from build123d import *

# Parameters (mm, degrees)
F1_W     = 43.7
F1_H     = 42.4
F1_R     = 1.5
F1_W_2   = 5
F1_H_2   = 4.4
F2_DEPTH = 1
F3_SIZE  = 0.99999
F4_DEPTH = 1
F5_W     = 19
F5_H     = 1
F6_DEPTH = 12


# Not quite as in the source:
# - a fillet or chamfer is up to 0.001 mm smaller than in the source, because OpenCascade refuses the exact size


with BuildPart() as f2:
    # F1 (on face) → F2 (new body)
    with BuildSketch(Plane.XY):
        with Locations((-38.7602308843, 29.1194021702)):
            Rectangle(F1_W, F1_H)
        with Locations((-53.3102308843, 12.9194021702)):
            Circle(F1_R, mode=Mode.SUBTRACT)
        with Locations((-48.3102308843, 13.1194021702)):
            Circle(F1_R, mode=Mode.SUBTRACT)
        with Locations((-41.9102308843, 33.1194021702)):
            Rectangle(F1_W_2, F1_H_2, mode=Mode.SUBTRACT)
        with Locations((-30.4102308843, 38.3194021702)):
            Circle(F1_R, mode=Mode.SUBTRACT)
        with BuildLine():
            ThreePointArc((-26.4145926142, 28.1194021702), (-29.3713070947, 29.1194021702), (-26.4145926142, 30.1194021702))
            Line((-26.4145926142, 30.1194021702), (-23.1138560921, 30.1194021702))
            Line((-23.1138560921, 30.1194021702), (-23.1138560921, 28.1194021702))
            Line((-23.1138560921, 28.1194021702), (-26.4145926142, 28.1194021702))
        make_face(mode=Mode.SUBTRACT)
        with Locations((-21.9102308843, 45.3194021702)):
            Circle(F1_R, mode=Mode.SUBTRACT)
    extrude(amount=F2_DEPTH)

    # F3 (size 1 in the source; OpenCascade refuses exactly that, so slightly less here)
    f3_edges = [f2.edges().sort_by_distance(p)[0] for p in [
        (-23.410231, 45.319402, 1),
        (-54.810231, 12.919402, 1),
    ]]
    chamfer(f3_edges, length=F3_SIZE)

    # F4 (add): a face of the model
    f4_faces = [f2.faces().sort_by_distance(p)[0] for p in [
        (-38.8442562914, 29.0967487251, 1),
    ]]
    extrude(f4_faces, amount=F4_DEPTH)

    # F5 (on face) → F6 (join)
    with BuildSketch(Plane.XY):
        with Locations((-28.9102308843, 8.4194021702)):
            Rectangle(F5_W, F5_H)
    extrude(amount=-F6_DEPTH)


solid = f2.part
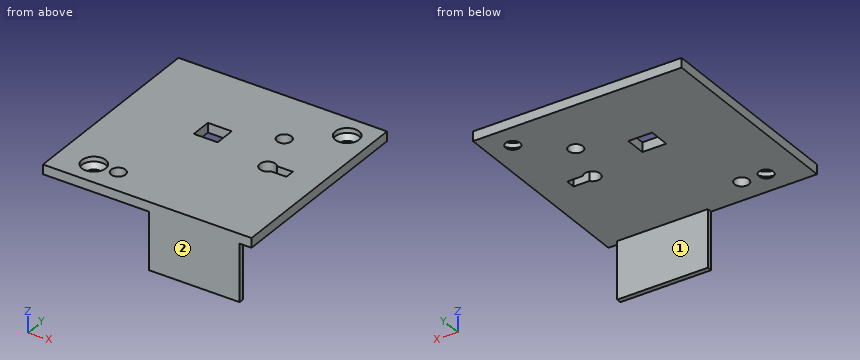
Geometry check sheet. Reference: the model listing, model coordinates, mm. Face numbers are marked on the shaded views. A direction names the side the tool comes from. Round coordinates to 2 decimals unless told otherwise and drop trailing zeros. Loops run counter-clockwise (first coordinate to the right, second up) from the corner with the lowest first, then second, coordinate; pieces in that order, holes last. Notation, with made-up numbers: (64.5, -40) -> (91.5, -40) arc R16 ccw to (91.5, -17) -> close; hole circle Ø10 at (67, -34). An arc over 180 degrees is marked (long way). Answer as a JSON object with one key per item and string values. Group by question number.
Item 1: Cross-section at D-D, the plane z = -6. Record the cut outline in (x, y), plus the area to 3 significant figures.
Item 2: Thickness scan on line 1 along Z through (x, y) = (-47, 43); line 2 along Y through (x, z) = (-24, -3.25); line 3 along Y through (x, z) = (-25, 1.5). Record the ranges inside material, lowest first.
Item 3: Cross-section at A-A, the plane y = 34. Record the cut outline in (x, z).
Item 4: Cross-section at C-C, the plane y = 29. Record the cut outline in (x, z), plus the area to 3 significant figures.
Item 5: Cross-section at B-B, the plane x = -36. Record the cut outline in (y, z), plus the area to 3 significant figures.
Item 6: Set-up check for the marked faces 1 and 2: record each of +Z, -Z, +X, -X, +Y, -Y from which the full face is reachable in a straight line by a thin tool's end or side.
Item 7: Depth check by flat-ended pin: pin 1 Ø12.5 at (x, y) = (-38, 34) entering from -Z; pin 2 Ø0.5 at (y, z) = (8.5, -6) entering from -X; pin 3 Ø1.1 at (y, z) = (8.5, -4) entering from +X. Enter the tip coordinate at first touch or a pass-through.
Determined:
{
 "1": {"outline": "(-38.41, 7.92) -> (-19.41, 7.92) -> (-19.41, 8.92) -> (-38.41, 8.92) -> close", "area": "19.0 mm²"},
 "2": {"line 1": "z = 0 to 2", "line 2": "y = 7.92 to 8.92", "line 3": "y = 7.92 to 28.12, 30.12 to 50.32"},
 "3": {"outline": "(-60.61, 0) -> (-44.41, 0) -> (-44.41, 2) -> (-60.61, 2) -> close; (-39.41, 0) -> (-16.91, 0) -> (-16.91, 2) -> (-39.41, 2) -> close"},
 "4": {"outline": "(-60.61, 0) -> (-29.37, 0) -> (-29.37, 2) -> (-60.61, 2) -> close; (-23.11, 0) -> (-16.91, 0) -> (-16.91, 2) -> (-23.11, 2) -> close", "area": "74.9 mm²"},
 "5": {"outline": "(7.92, -12) -> (8.92, -12) -> (8.92, 0) -> (50.32, 0) -> (50.32, 2) -> (7.92, 2) -> close", "area": "96.8 mm²"},
 "6": {"face 1": "-Z, +X, -X, +Y", "face 2": "+Z, -Z, +X, -X, -Y"},
 "7": {"pin 1": "stops at z = 0", "pin 2": "stops at x = -38.41", "pin 3": "stops at x = -19.41"}
}
